```python
from build123d import *

# Parameters (mm, degrees)
SKETCH_W        = 950
SKETCH_H        = 850
PAD_DEPTH       = 150
SKETCH002_W     = 200
SKETCH002_H     = 310
POCKET_DEPTH    = 20
SKETCH003_W     = 400
SKETCH003_H     = 850
POCKET001_DEPTH = 20
POCKET002_DEPTH = 150.001


with BuildPart() as part:
    # Sketch → Pad (new body)
    with BuildSketch(Plane.XY):
        with Locations((475, 425)):
            Rectangle(SKETCH_W, SKETCH_H)
    extrude(amount=PAD_DEPTH)

    # Sketch002 (on Face6 of Pad) → Pocket (cut)
    with BuildSketch(Plane.XY.offset(150)):
        with Locations((100, 695)):
            Rectangle(SKETCH002_W, SKETCH002_H)
        with Locations((850, 695)):
            Rectangle(SKETCH002_W, SKETCH002_H)
    extrude(amount=-POCKET_DEPTH, mode=Mode.SUBTRACT)

    # Sketch003 (on Face5 of Pocket) → Pocket001 (cut)
    with BuildSketch(Plane.XY.offset(150)):
        with Locations((475, 425)):
            Rectangle(SKETCH003_W, SKETCH003_H)
    extrude(amount=-POCKET001_DEPTH, mode=Mode.SUBTRACT)

    # Sketch004 (on Face4 of Pocket001) → Pocket002 (cut, through all)
    with BuildSketch(Plane.XY.offset(150)):
        Polygon((0, 510), (175, 335), (175, 0), (0, 0), align=None)
        Polygon((950, 510), (775, 335), (775, 0), (950, 0), align=None)
    extrude(amount=-POCKET002_DEPTH, mode=Mode.SUBTRACT)


solid = part.part
```
Source: CAD feature listing. Evaluate the final solid. Frame: model axes, mm. A direction names the side the tool comes from. Round coordinates to 2 decimals unless told otherwise and drop trailing zeros. Write each loop counter-clockwise with the first axis right and the second up, starting at its lowest first coordinate (ties: lowest second). Pieces come first, ordered by that corner, then holes. Notation, with made-up numbers: M 2,65.25 L 59,65.25 A16 cw 59,91.25 Z; hole C 40.25,89 d10. An arc over 180 degrees is marked long. Answer as a JSON object with one key per item and string values. Group by question number.
(1) Section query A-A on y = 203. Output: boundary loops of the cut face in (x, z), then the cut area to 3 significant figures.
(2) Section query C-C on x = 408. Output: boundary loops of the cut face in (y, z).
(3) Mould query, pull axis X, two halves, no side actions, for faces 1 (the flat face through (472, 431, 130)), 2 (the flat face through (197, 431, 150)), 3 (the flat face through (950, 678, 74)), 4 (the flat face through (175, 170, 76)). Classes: +X half, -X half, draft (parallel to the pull), parting line (faces both ways), or undercut.
(4) First-contact query: pin 1 (3 mm diameter, centred on x = 823.5, y = 666.5, fed in from +Z); pin 2 (22 mm diameter, centred on y = 445.5, z = 145, fed in from +X); pin 3 (16 mm diameter, centred on y = 675.5, z = 138.5, fed in from +X). Flat tips, straight axial feed; report the tip coordinate or a pass-through.
(5) Section query B-B on z = 92. Output: boundary loops of the cut face in (x, y).
(6) Section query D-D on y = 605. Output: boundary loops of the cut face in (x, z).
(7) Reachability of faces 5 (the flat face through (0, 678, 74)), 6 (the flat face through (749, 431, 150)), 7 (the flat face through (675, 419, 140)), 8 (the flat face through (849, 697, 130)), 9 (the flat face through (200, 693, 140)) from +Z, -Z, +X, -X, +Y, -Y: full face, straight path, thin tool, end or side. Return the list, or none.
(8) Ray query, line 1 (X direction, y = 811, z = 142); line 2 (X direction, y = 249.5, z = 29.5); line 3 (Z direction, x = 849, y = 788). Return the intervals inside material, ascending. Write a range as [from, to].
Computed values:
{
 "1": {"outline": "M 175,0 L 775,0 L 775,150 L 675,150 L 675,130 L 275,130 L 275,150 L 175,150 Z", "area": "82,000 mm^2"},
 "2": {"outline": "M 0,0 L 850,0 L 850,130 L 0,130 Z"},
 "3": {"face 1": "undercut", "face 2": "draft", "face 3": "+X half", "face 4": "-X half"},
 "4": {"pin 1": "z = 130", "pin 2": "x = 896.5", "pin 3": "x = 750"},
 "5": {"outline": "M 0,510 L 175,335 L 175,0 L 775,0 L 775,335 L 950,510 L 950,850 L 0,850 Z"},
 "6": {"outline": "M 0,0 L 950,0 L 950,130 L 750,130 L 750,150 L 675,150 L 675,130 L 275,130 L 275,150 L 200,150 L 200,130 L 0,130 Z"},
 "7": {"face 5": "+Z, -Z, -X, +Y, -Y", "face 6": "+Z, +X, -X, +Y, -Y", "face 7": "+Z, +Y, -Y", "face 8": "+Z, +X, +Y", "face 9": "+Z, -X, +Y"},
 "8": {"line 1": "[200, 275], [675, 750]", "line 2": "[175, 775]", "line 3": "[0, 130]"}
}
